Geometry: final body of the model. Coordinates: model frame, mm. Face numbers are marked on the shaded views. A direction names the side the tool comes from. Coordinates: 2 decimals unless noted, no trailing zeros. Loops run counter-clockwise (first coordinate to the right, second up) from the corner with the lowest first, then second, coordinate; pieces in that order, holes last. Notation, with made-up numbers: (46.5, -29) - (85.5, -29) arc R24 cw to (85.5, -5) - close; hole circle Ø10 at (11.25, 12.5). An arc over 180 degrees is marked (long way). Put each result on its own line as item: value. Start each with the question number.
1) Draft query along Y for the marked faces 5, 6 and 7. Return one class per face: +Y half, -Y half, draft (parallel to the pull), parting line (faces both ways), or undercut.
2) Material intervals for line 1 along Y through (x, z) = (28, 6.5); line 2 along Y through (x, z) = (30.5, 5); line 3 along Y through (x, z) = (33, -7), sorted ascending. Write a range as from..to.
3) Section C-C on y = 41.75. Output: boundary loops of the cut face in (x, z).
4) Section B-B on x = 45.75. Output: boundary loops of the cut face in (y, z), and give its area (3 significant figures).
5) Reachability of the marked faces 1, 2, 3 and 4 from +Z, -Z, +X, -X, +Y, -Y: full face, straight path, thin tool, end or side. Return the list, or none.
6) Section A-A on y = 37.25. Output: boundary loops of the cut face in (x, z).
7) Contact query for flat-ended pins moving along their axis: pin 1 Ø2 at (y, z) = (29, -6.5) entering from +X; pin 2 Ø0.9 at (y, z) = (24, 3.5) entering from +X; pin 3 Ø0.9 at (y, z) = (24, -0.5) entering from -X. Output: stop coordinate, or through.
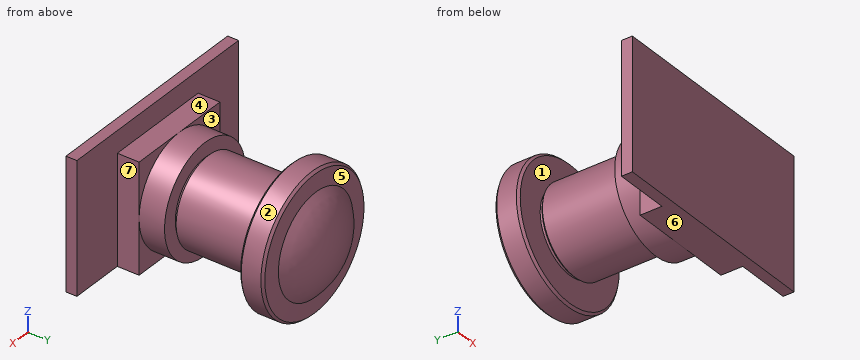
```python
from build123d import *

# Parameters (mm, degrees)
SCALE1_SCALE        = 0.268090154
SKETCH2_R           = 7.5
BOSS_EXTRUDE1_DEPTH = 3.5
SKETCH3_W           = 15
SKETCH3_H           = 15
BOSS_EXTRUDE2_DEPTH = 3
SKETCH4_W           = 30
SKETCH4_H           = 18
BOSS_EXTRUDE3_DEPTH = 1.5


with BuildPart() as part:
    # Model → Revolve1 (revolve)
    with BuildSketch(Plane.XY):
        with BuildLine():
            Line((35.565588, 69.903749404), (35.565588, 2.41570256))
            Line((35.565588, 2.41570256), (15.0702518, 2.41570256))
            Line((15.0702518, 2.41570256), (13.1823206, 4.2595038))
            Line((13.1823206, 4.2595038), (13.1823206, 43.648122))
            Line((13.1823206, 43.648122), (14.1483334, 44.569888))
            Line((14.1483334, 44.569888), (15.0702518, 44.569888))
            Line((15.0702518, 44.569888), (15.0702518, 46.238668))
            Line((15.0702518, 46.238668), (2.9572712, 46.238668))
            Line((2.9572712, 46.238668), (1.28984502, 46.238668))
            Line((1.28984502, 46.238668), (0.148828252, 47.38116))
            Line((0.148828252, 47.38116), (0.148828252, 57.436766))
            Line((0.148828252, 57.436766), (1.24574554, 58.665872))
            Line((1.24574554, 58.665872), (9.701542865, 59.330571423))
            ThreePointArc((9.701542865, 59.330571423), (21.589655561, 67.170766536), (35.565588, 69.903749404))
        make_face()
    revolve(axis=Axis((35.565588, 69.903749404, 0), (0, -1, 0)))


with BuildPart() as part_1:
    # Scale1: scaled about (35.565588, 38.752959179, 0)
    add(part.part.scale(SCALE1_SCALE).moved(Location((26.030804028, 28.363672377, 0))))

    # Sketch2 → Boss-Extrude1 (add)
    with BuildSketch(Plane.XZ.offset(-29.011298449)):
        with Locations((35.565588, 0)):
            Circle(SKETCH2_R)
    extrude(amount=BOSS_EXTRUDE1_DEPTH)

    # Sketch3 → Boss-Extrude2 (add)
    with BuildSketch(Plane.XZ.offset(-25.511298449)):
        with Locations((35.565588, 0)):
            Rectangle(SKETCH3_W, SKETCH3_H)
    extrude(amount=BOSS_EXTRUDE2_DEPTH)

    # Sketch4 → Boss-Extrude3 (add)
    with BuildSketch(Plane.XZ.offset(-22.511298449)):
        with Locations((35.565588, 1.5)):
            Rectangle(SKETCH4_W, SKETCH4_H)
    extrude(amount=BOSS_EXTRUDE3_DEPTH)


solid = part_1.part
```
Answer block:
1. face 5: +Y half
1. face 6: draft
1. face 7: undercut
2. line 1: y = 21.01..22.51
2. line 2: y = 21.01..29.01, 40.76..44.26
2. line 3: y = 21.01..29.01, 40.76..44.23
3. outline: circle Ø18.99 at (35.57, 0)
4. outline: (21.01, -7.5) - (22.51, -7.5) - (22.51, 10.5) - (21.01, 10.5) - close
4. area: 27.0 mm²
5. face 1: none
5. face 2: +Y
5. face 3: +Z, -X
5. face 4: +Z, +X, -X
6. outline: circle Ø12 at (35.57, 0)
7. pin 1: stops at x = 40.66
7. pin 2: stops at x = 43.07
7. pin 3: stops at x = 28.07
